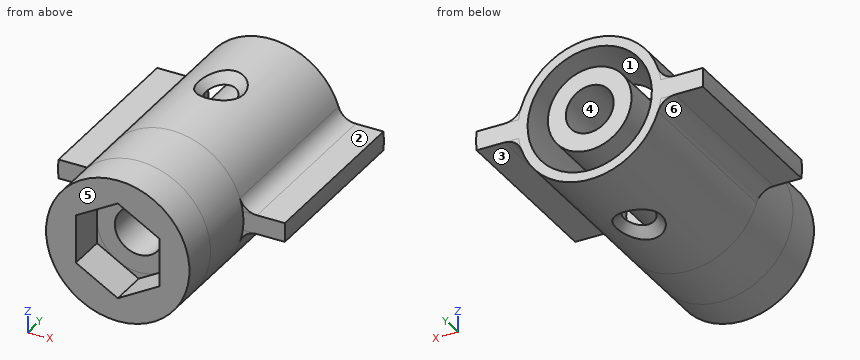
```python
from build123d import *

# Parameters (mm, degrees)
SKETCH1_R           = 3.5
SKETCH1_R_2         = 2
BOSS_EXTRUDE1_DEPTH = 20
SKETCH1_3_R         = 6
BOSS_EXTRUDE2_DEPTH = 3.2
SKETCH1_4_R         = 6
BOSS_EXTRUDE3_DEPTH = 5
SKETCH2_R           = 5.2
BOSS_EXTRUDE4_DEPTH = 15
CIRPATTERN1_COUNT   = 2
FILLET1_R           = 1.5


with BuildPart() as part:
    # Sketch1 → Boss-Extrude1 (new body)
    with BuildSketch(Plane(origin=(0, 0, 0), x_dir=(1, 0, 0), z_dir=(0, 1, 0))):
        with Locations(Location((0, 0, 0), (0, 0, 270))):
            Circle(SKETCH1_R)
        with Locations(Location((0, 0, 0), (0, 0, 270))):
            Circle(SKETCH1_R_2, mode=Mode.SUBTRACT)
    extrude(amount=BOSS_EXTRUDE1_DEPTH)



with BuildPart() as body_2:
    # Sketch1<3> → Boss-Extrude2 (new body)
    with BuildSketch(Plane(origin=(0, 0, 0), x_dir=(1, 0, 0), z_dir=(0, 1, 0))):
        with Locations(Location((0, 0, 0), (0, 0, 270))):
            Circle(SKETCH1_3_R)
        Polygon((0, -4.041451884), (3.5, -2.020725942), (3.5, 2.020725942), (0, 4.041451884), (-3.5, 2.020725942), (-3.5, -2.020725942), align=None, mode=Mode.SUBTRACT)
    extrude(amount=-BOSS_EXTRUDE2_DEPTH)


with BuildPart() as part_1:
    add(part.part)

    add(body_2.part)  # Boss-Extrude3 merges body 2
    # Sketch1<4> → Boss-Extrude3 (add)
    # profile 1 of 7: a face of its own
    with BuildSketch(Plane(origin=(0, 0, 0), x_dir=(1, 0, 0), z_dir=(0, 1, 0))):
        with Locations(Location((0, 0, 0), (0, 0, 270))):
            Circle(SKETCH1_4_R)
        Polygon((0, -4.041451884), (3.5, -2.020725942), (3.5, 2.020725942), (0, 4.041451884), (-3.5, 2.020725942), (-3.5, -2.020725942), align=None, mode=Mode.SUBTRACT)
    # profile 2 of 7: a face of its own
    with BuildSketch(Plane(origin=(0, 0, 0), x_dir=(1, 0, 0), z_dir=(0, 1, 0))):
        with BuildLine():
            ThreePointArc((-1.749999906, 3.031088968), (8.8e-08, 3.5), (1.750000057, 3.03108888))
            Line((1.750000057, 3.03108888), (0, 4.041451884))
            Line((0, 4.041451884), (-1.749999906, 3.031088968))
        make_face()
    # profile 3 of 7: a face of its own
    with BuildSketch(Plane(origin=(0, 0, 0), x_dir=(1, 0, 0), z_dir=(0, 1, 0))):
        with BuildLine():
            ThreePointArc((1.750000057, 3.03108888), (3.03108893, 1.749999971), (3.5, 0))
            Line((3.5, 0), (3.5, 2.020725942))
            Line((3.5, 2.020725942), (1.750000057, 3.03108888))
        make_face()
    # profile 4 of 7: a face of its own
    with BuildSketch(Plane(origin=(0, 0, 0), x_dir=(1, 0, 0), z_dir=(0, 1, 0))):
        with BuildLine():
            Line((1.750000074, -3.03108887), (3.5, -2.020725942))
            Line((3.5, -2.020725942), (3.5, 0))
            ThreePointArc((3.5, 0), (3.031088935, -1.749999963), (1.750000074, -3.03108887))
        make_face()
    # profile 5 of 7: a face of its own
    with BuildSketch(Plane(origin=(0, 0, 0), x_dir=(1, 0, 0), z_dir=(0, 1, 0))):
        with BuildLine():
            Line((0, -4.041451884), (1.750000074, -3.03108887))
            ThreePointArc((1.750000074, -3.03108887), (5.1e-08, -3.5), (-1.749999986, -3.031088921))
            Line((-1.749999986, -3.031088921), (0, -4.041451884))
        make_face()
    # profile 6 of 7: a face of its own
    with BuildSketch(Plane(origin=(0, 0, 0), x_dir=(1, 0, 0), z_dir=(0, 1, 0))):
        with BuildLine():
            Line((-3.5, -2.020725942), (-1.749999986, -3.031088921))
            ThreePointArc((-1.749999986, -3.031088921), (-3.031088909, -1.750000007), (-3.5, 0))
            Line((-3.5, 0), (-3.5, -2.020725942))
        make_face()
    # profile 7 of 7: a face of its own
    with BuildSketch(Plane(origin=(0, 0, 0), x_dir=(1, 0, 0), z_dir=(0, 1, 0))):
        with BuildLine():
            ThreePointArc((-3.5, 0), (-3.031088886, 1.750000047), (-1.749999906, 3.031088968))
            Line((-1.749999906, 3.031088968), (-3.5, 2.020725942))
            Line((-3.5, 2.020725942), (-3.5, 0))
        make_face()
    extrude(amount=BOSS_EXTRUDE3_DEPTH)

    # Sketch2 → Boss-Extrude4 (add)
    with BuildSketch(Plane(origin=(0, 5, 0), x_dir=(1, 0, 0), z_dir=(0, 1, 0))):
        with BuildLine():
            Line((-9.46625586, -0.8), (-5.946427499, -0.8))
            ThreePointArc((-5.946427499, -0.8), (0, -6), (5.946427499, -0.8))
            Line((5.946427499, -0.8), (9.46625586, -0.8))
            ThreePointArc((9.46625586, -0.8), (9.5, 0), (9.46625586, 0.8))
            Line((9.46625586, 0.8), (5.946427499, 0.8))
            ThreePointArc((5.946427499, 0.8), (0, 6), (-5.946427499, 0.8))
            Line((-5.946427499, 0.8), (-9.46625586, 0.8))
            ThreePointArc((-9.46625586, 0.8), (-9.5, 0), (-9.46625586, -0.8))
        make_face()
        with Locations(Location((0, 0, 0), (0, 0, 270))):
            Circle(SKETCH2_R, mode=Mode.SUBTRACT)
    extrude(amount=BOSS_EXTRUDE4_DEPTH)

    # Sketch5 → CSK for M2 Flat Head Machine Screw1 (revolve, cut)
    with BuildSketch(Plane(origin=(0, 12.5, -6), x_dir=(0, 1, 0), z_dir=(1, 0, 0))):
        Polygon((0, 0), (0, 5), (1.2, 4.278967257), (1.2, 1), (2.2, 0), align=None)
    csk_for_m2_flat_head_machine_screw1 = revolve(axis=Axis((0, 12.5, -12.35), (0, 0, 1)), mode=Mode.SUBTRACT)

    # CirPattern1: CSK for M2 Flat Head Machine Screw1 ×2 about axis
    cirpattern1_axis = Axis((0, 5, 0), (0, -1, 0))
    for i in range(1, CIRPATTERN1_COUNT):
        add(csk_for_m2_flat_head_machine_screw1.rotate(cirpattern1_axis, i * 360 / CIRPATTERN1_COUNT), mode=Mode.SUBTRACT)

    # Fillet1
    # the kernel refuses this fillet: 1.5 mm, written as the material it adds along each edge
    with BuildSketch(Plane(origin=(-5.946427499, 5, 0.8), x_dir=(-1, 0, 0), z_dir=(0, 1, 0)), Plane(origin=(5.946427499, 5, -0.8), x_dir=(1, 0, 0), z_dir=(0, 1, 0))) as fillet1_piece_1:
        with BuildLine():
            CenterArc((1.19219982, 1.5), FILLET1_R, 197.858462698, 72.141537302)
            ThreePointArc((-0.235525644, 1.04), (-0.094613086, 0.52524265), (0, 0))
            Line((0, 0), (1.19219982, 0))
        make_face()
    extrude(amount=15)
    with BuildSketch(Plane(origin=(5.946427499, 5, 0.8), x_dir=(1, 0, 0), z_dir=(0, 1, 0)), Plane(origin=(-5.946427499, 5, -0.8), x_dir=(-1, 0, 0), z_dir=(0, 1, 0))) as fillet1_piece_2:
        with BuildLine():
            CenterArc((1.19219982, -1.5), FILLET1_R, 90, 72.141537302)
            ThreePointArc((-0.235525644, -1.04), (-0.094613086, -0.52524265), (0, 0))
            Line((0, 0), (1.19219982, 0))
        make_face()
    extrude(amount=15)


solid = part_1.part
```
CAD build for the part. Positions are in the model's coordinates, mm. Face numbers are marked on the shaded views. A direction names the side the tool comes from. Round coordinates to 2 decimals unless told otherwise and drop trailing zeros. Write each loop counter-clockwise with the first axis right and the second up, starting at its lowest first coordinate (ties: lowest second). Pieces come first, ordered by that corner, then holes.
Item 1: Band-saw the part on C-C on y = 12.5. Give the number of separate pieces and of enclosed holes in the cut face, then the cut area to 3 significant figures.
Filled in:
separate pieces: 4
enclosed holes: 0
area: 53.8 mm2
Item 2: Band-saw the part on B-B on y = -1. Write the cut outline in (x, z), then the cut area to 3 significant figures.
Filled in:
outline: circle Ø12 at (0, 0); hole (-3.5, -2.02) - (0, -4.04) - (3.5, -2.02) - (3.5, 2.02) - (0, 4.04) - (-3.5, 2.02) - close
area: 70.7 mm2
Item 3: Drill centre lines: L1, parallel to Z at x = 0, y = 10.25; L2, parallel to X at y = 12.5, z = -2.65; L3, parallel to X at y = 13, z = 2.5. Where is each one in solid material? Low to high.
Filled in:
L1: z = -6 to -5.2, -3.5 to -2, 2 to 3.5, 5.2 to 6
L2: x = -5.38 to -4.47, -2.29 to -1.2, 1.2 to 2.29, 4.47 to 5.38
L3: x = -5.45 to -4.56, -2.45 to -1.09, 1.09 to 2.45, 4.56 to 5.45
Item 4: Tool access for the marked faces 1, 2 and 3: list every direction of +Z, -Z, +X, -X, +Y, -Y with a clear straight run to the whole face (end or side of a thin tool).
Filled in:
face 1: +Y
face 2: +Z, +X, +Y, -Y
face 3: -Z, +X, +Y, -Y
Item 5: Band-saw the part on A-A on y = 9. Write the cut outline in (x, z), then the cut area to 3 significant figures.
Filled in:
outline: (-9.47, -0.8) - (-7.14, -0.8) arc R1.5 cw to (-5.71, -1.84) arc R6 ccw to (5.71, -1.84) arc R1.5 cw to (7.14, -0.8) - (9.47, -0.8) arc R9.5 ccw to (9.47, 0.8) - (7.14, 0.8) arc R1.5 cw to (5.71, 1.84) arc R6 ccw to (-5.71, 1.84) arc R1.5 cw to (-7.14, 0.8) - (-9.47, 0.8) arc R9.5 ccw to start; circle Ø7 at (0, 0); hole circle Ø10.4 at (0, 0); hole circle Ø4 at (0, 0)
area: 66.3 mm2
Item 6: Mould opens along X. For the marked faces 4, 5 and 6 say: released by +X, released by -X, zero draft, split by the parting line, or undercut.
Filled in:
face 4: undercut
face 5: zero draft
face 6: released by -X
Item 7: Band-saw the part on D-D on x = -4.75. Write the cut outline in (y, z).
Filled in:
outline: (-3.2, -3.67) - (20, -3.67) - (20, -2.12) - (5, -2.12) - (5, 2.12) - (20, 2.12) - (20, 3.67) - (-3.2, 3.67) - close
Item 8: Drop flat-ended pins along their axis: pin 1 Ø1 at (y, z) = (14.5, 2) entering from -X; pin 2 Ø6 at (y, z) = (4.5, 4.5) entering from +X; pin 3 Ø1 at (y, z) = (13.5, -3.5) entering from -X; pin 4 Ø0.8 at (x, z) = (-6.5, -1.5) entering from -Y. Give the stop position or say it passes through.
Filled in:
pin 1: stops at x = -5.87
pin 2: stops at x = 5.84
pin 3: stops at x = -5.2
pin 4: passes through
